Could you check a few things on this model? Use its own coordinates, in mm. Give positions to 0.01 mm unless a question says otherwise; leave off trailing zeros. Write each loop counter-clockwise with the first axis right and the second up, starting at its lowest first coordinate (ties: lowest second). Pieces come first, ordered by that corner, then holes. Notation, with made-up numbers: (84, 19) -> (99, 19) arc R23 ccw to (99, 39) -> close; hole circle Ø2 at (23.5, 76). An arc over 180 degrees is marked (long way). Write item = value, one per line. Start each with the question number.
```python
from build123d import *

# Parameters (mm, degrees)
F0_W     = 500
F0_H     = 250
F1_DEPTH = 25
F2_R     = 50
F3_R     = 8
F4_DEPTH = 25.001


with BuildPart() as f1:
    # F0 (on Top) → F1 (new body)
    with BuildSketch(Plane.XY):
        Rectangle(F0_W, F0_H)
    extrude(amount=F1_DEPTH)

    # F2
    f2_edges = [f1.edges().sort_by_distance(p)[0] for p in [
        (-250, -125, 12.5),
        (250, -125, 12.5),
        (250, 125, 12.5),
        (-250, 125, 12.5),
    ]]
    fillet(f2_edges, radius=F2_R)

    # F3 (on face) → F4 (cut, through all)
    with BuildSketch(Plane.XY.offset(25)):
        Circle(F3_R)
    extrude(amount=-F4_DEPTH, mode=Mode.SUBTRACT)


solid = f1.part
```
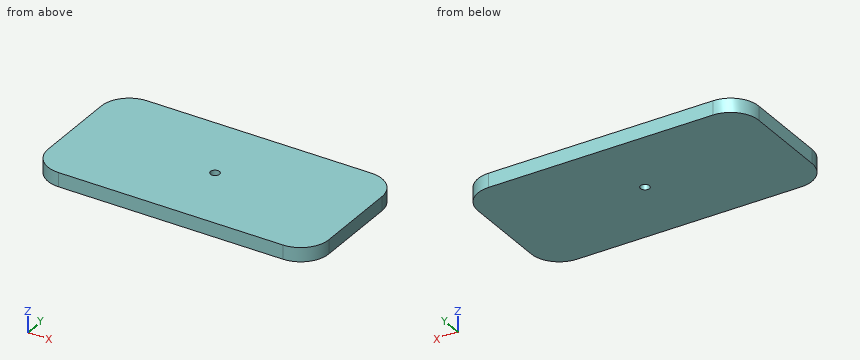
(1) If I drill on line 1 along Y through (x, z) = (0, 16.5); line 2 along X through (y, z) = (102, 23); line 3 along X through (y, z) = (-84, 13.75), over which ranges is the centre line in solid material (lowest first)? Write a range as from..to.
(2) Imagine slicing it at C-C (z = 19.25). Please give me the cut outline in (x, y), then the cut area to 3 significant figures.
(3) Imagine slicing it at B-B (x = 0). Please give me the cut outline in (y, z), then the cut area to 3 significant figures.
(4) Imagine slicing it at A-A (y = 0). Please give me the cut outline in (x, z), then the cut area to 3 significant figures.
Answers below:
q1.line_1 = -125..-8, 8..125
q1.line_2 = -242.08..242.08
q1.line_3 = -249.18..249.18
q2.outline = (-250, -75) arc R50 ccw to (-200, -125) -> (200, -125) arc R50 ccw to (250, -75) -> (250, 75) arc R50 ccw to (200, 125) -> (-200, 125) arc R50 ccw to (-250, 75) -> close; hole circle Ø16 at (0, 0)
q2.area = 123,000 mm^2
q3.outline = (-125, 0) -> (-8, 0) -> (-8, 25) -> (-125, 25) -> close; (8, 0) -> (125, 0) -> (125, 25) -> (8, 25) -> close
q3.area = 5,850 mm^2
q4.outline = (-250, 0) -> (-8, 0) -> (-8, 25) -> (-250, 25) -> close; (8, 0) -> (250, 0) -> (250, 25) -> (8, 25) -> close
q4.area = 12,100 mm^2
